Could you check a few things on this model? Use its own coordinates, in mm. A direction names the side the tool comes from. Coordinates: 2 decimals unless noted, no trailing zeros. Loops run counter-clockwise (first coordinate to the right, second up) from the corner with the lowest first, then second, coordinate; pieces in that order, holes last.
from build123d import *

# Parameters (mm, degrees)
SKETCH1_W           = 165
SKETCH1_H           = 20
SKETCH1_R           = 1.7
BOSS_EXTRUDE1_DEPTH = 6.35
CUT_EXTRUDE2_DEPTH  = 3.35
CUT_EXTRUDE3_DEPTH  = 3


with BuildPart() as part:
    # Sketch1 → Boss-Extrude1 (new body)
    with BuildSketch(Plane(origin=(0, 0, 0), x_dir=(-1, 0, 0), z_dir=(0, 0, 1))):
        with Locations((52.952306935, 12.575384489)):
            Rectangle(SKETCH1_W, SKETCH1_H)
        with Locations(Location((120.452306935, 12.575384489, 0), (0, 0, 180))):
            Circle(SKETCH1_R, mode=Mode.SUBTRACT)
        with Locations(Location((-14.547693065, 12.575384489, 0), (0, 0, 180))):
            Circle(SKETCH1_R, mode=Mode.SUBTRACT)
    extrude(amount=BOSS_EXTRUDE1_DEPTH)

    # Sketch3 → Cut-Extrude2 (cut)
    with BuildSketch(Plane(origin=(0, 0, 0), x_dir=(-1, 0, 0), z_dir=(0, 0, -1))):
        with BuildLine():
            Line((56.502306935, -16.125384489), (49.402306935, -16.125384489))
            ThreePointArc((49.402306935, -16.125384489), (45.852306935, -12.575384489), (49.402306935, -9.025384489))
            Line((49.402306935, -9.025384489), (56.502306935, -9.025384489))
            ThreePointArc((56.502306935, -9.025384489), (60.052306935, -12.575384489), (56.502306935, -16.125384489))
        make_face()
        with BuildLine():
            Line((101.502306935, -16.125384489), (94.402306935, -16.125384489))
            ThreePointArc((94.402306935, -16.125384489), (90.852306935, -12.575384489), (94.402306935, -9.025384489))
            Line((94.402306935, -9.025384489), (101.502306935, -9.025384489))
            ThreePointArc((101.502306935, -9.025384489), (105.052306935, -12.575384489), (101.502306935, -16.125384489))
        make_face()
        with BuildLine():
            Line((11.502306935, -16.125384489), (4.402306935, -16.125384489))
            ThreePointArc((4.402306935, -16.125384489), (0.852306935, -12.575384489), (4.402306935, -9.025384489))
            Line((4.402306935, -9.025384489), (11.502306935, -9.025384489))
            ThreePointArc((11.502306935, -9.025384489), (15.052306935, -12.575384489), (11.502306935, -16.125384489))
        make_face()
    extrude(amount=-CUT_EXTRUDE2_DEPTH, mode=Mode.SUBTRACT)

    # Sketch4 → Cut-Extrude3 (cut)
    with BuildSketch(Plane(origin=(0, 0, 3.35), x_dir=(-1, 0, 0), z_dir=(0, 0, -1))):
        with BuildLine():
            ThreePointArc((9.952306935, -12.575384489), (9.366520498, -11.161170927), (7.952306935, -10.575384489))
            Line((7.952306935, -10.575384489), (7.952306935, -14.575384489))
            ThreePointArc((7.952306935, -14.575384489), (9.366520498, -13.989598052), (9.952306935, -12.575384489))
        make_face()
        with BuildLine():
            Line((7.952306935, -14.575384489), (7.952306935, -10.575384489))
            ThreePointArc((7.952306935, -10.575384489), (5.952306935, -12.575384489), (7.952306935, -14.575384489))
        make_face()
        with BuildLine():
            ThreePointArc((52.952306935, -10.575384489), (50.952306935, -12.575384489), (52.952306935, -14.575384489))
            Line((52.952306935, -14.575384489), (52.952306935, -10.575384489))
        make_face()
        with BuildLine():
            Line((52.952306935, -10.575384489), (52.952306935, -14.575384489))
            ThreePointArc((52.952306935, -14.575384489), (54.366520498, -13.989598052), (54.952306935, -12.575384489))
            ThreePointArc((54.952306935, -12.575384489), (54.366520498, -11.161170927), (52.952306935, -10.575384489))
        make_face()
        with BuildLine():
            ThreePointArc((99.952306935, -12.575384489), (99.366520498, -11.161170927), (97.952306935, -10.575384489))
            Line((97.952306935, -10.575384489), (97.952306935, -14.575384489))
            ThreePointArc((97.952306935, -14.575384489), (99.366520498, -13.989598052), (99.952306935, -12.575384489))
        make_face()
        with BuildLine():
            Line((97.952306935, -14.575384489), (97.952306935, -10.575384489))
            ThreePointArc((97.952306935, -10.575384489), (95.952306935, -12.575384489), (97.952306935, -14.575384489))
        make_face()
    extrude(amount=-CUT_EXTRUDE3_DEPTH, mode=Mode.SUBTRACT)


solid = part.part
(1) We'd pull the mould along X, two halves only. Please class faces 1 (the face through (-52, -10, 6.35)), 2 (the face through (-98, -16.125, 2)), 3 (the face through (29.548, -12, 3)): +X half, -X half, draft (parallel to the pull), parting line (faces both ways), or undercut.
Answers:
face 1: draft
face 2: undercut
face 3: +X half
(2) I need wall thicknesses on probe 1 along X at (y, z) = (-12.5, 3.25); probe 2 along Y at (x, z) = (-7.5, 2.75); probe 3 along X at (y, z) = (-9.75, 1.5). Which ranges of each line are inside material? Lowest first, please.
Answers:
probe 1: x = -135.45 to -122.15, -118.75 to -105.05, -90.85 to -60.05, -45.85 to -15.05, -0.85 to 12.85, 16.25 to 29.55
probe 2: y = -22.58 to -16.13, -9.03 to -2.58
probe 3: x = -135.45 to -103.65, -92.25 to -58.65, -47.25 to -13.65, -2.25 to 29.55
(3) Imagine slicing it at A-A, the plane z = 5. Write out the boundary of the cut face in (x, y).
Answers:
outline: (-135.45, -22.58) - (29.55, -22.58) - (29.55, -2.58) - (-135.45, -2.58) - close; hole circle Ø3.4 at (-120.45, -12.58); hole circle Ø4 at (-97.95, -12.58); hole circle Ø4 at (-52.95, -12.58); hole circle Ø4 at (-7.95, -12.58); hole circle Ø3.4 at (14.55, -12.58)
(4) Which directions (+Z, -Z, +X, -X, +Y, -Y) give clear straight access to the entire face, cutting with the end or side of a thin tool? Please do faces 4 (the face through (-51, -14, 3.35)), 5 (the face through (-119.54, -11.14, 3.13)).
Answers:
face 4: -Z
face 5: +Z, -Z
(5) For pin 1 (3.5 mm diameter, centred on x = -55.5, y = -12, fed in from -Z), with a flat end and sliding along its axis, tell me the tip position at first contact or that it passes through.
Answers:
pin 1: stops at z = 3.35
(6) Imagine slicing it at B-B, the plane x = -47.5. Write out the boundary of the cut face in (y, z), and give its area (3 significant figures).
Answers:
outline: (-22.58, 0) - (-15.57, 0) - (-15.57, 3.35) - (-9.58, 3.35) - (-9.58, 0) - (-2.58, 0) - (-2.58, 6.35) - (-22.58, 6.35) - close
area: 107 mm2
